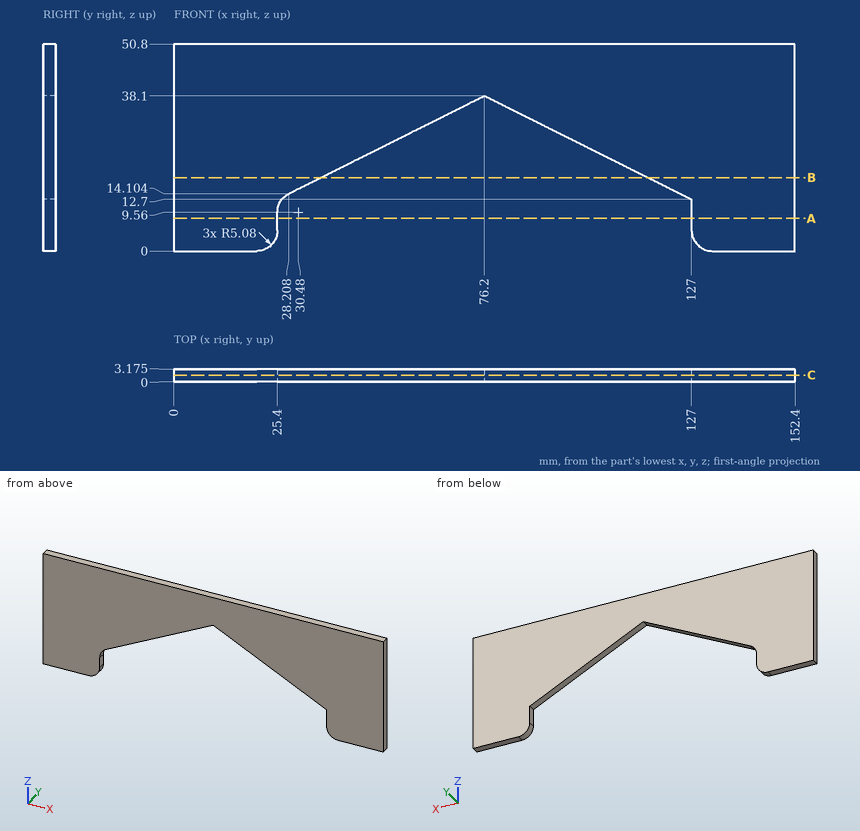
Design review of the part shown in the three views and the two pictorial views. Dimensions are in mm from the part's minimum x, y and z. Give positions to 0.01 mm unless a question says otherwise; leave off trailing zeros. Write each loop counter-clockwise with the first axis right and the second up, starting at its lowest first coordinate (ties: lowest second). Pieces come first, ordered by that corner, then holes. Notation, with made-up numbers: (53.5, 73) -> (82.5, 73) arc R15 ccw to (82.5, 83) -> close; hole circle Ø10 at (38.25, 45.25). An arc over 180 degrees is marked (long way). Answer in a Markdown table with one row per item.
1) Add section A-A on z = 8. State the section outline as (x, y) points (1 decimal).
Worked answers:
| item | result |
|---|---|
| outline | (0, 0) -> (25.4, 0) -> (25.4, 3.2) -> (0, 3.2) -> close; (127, 0) -> (152.4, 0) -> (152.4, 3.2) -> (127, 3.2) -> close |
2) Clearance check with a flat-ended pin moving along its axis: P1, Ø10, axis at x = 48, z = 19, coming from the +Y side (3 decimals). State where the tip first meets the part, or that it passes through.
Worked answers:
| item | result |
|---|---|
| P1 | y = 3.175 |
3) Add section B-B on z = 18. State the section outline as (x, y) points (1 decimal).
Worked answers:
| item | result |
|---|---|
| outline | (0, 0) -> (36, 0) -> (36, 3.2) -> (0, 3.2) -> close; (116.4, 0) -> (152.4, 0) -> (152.4, 3.2) -> (116.4, 3.2) -> close |
4) For L1, parallel to X at y = 0.5, z = 10; L2, parallel to X at y = 1.45, z = 23; L3, parallel to Z at x = 113.5, y = 2.7, list the stretches that pass through material, from the lowest coordinate up. Write a range as [from, to].
Worked answers:
| item | result |
|---|---|
| L1 | [0, 25.42], [127, 152.4] |
| L2 | [0, 46], [106.4, 152.4] |
| L3 | [19.45, 50.8] |
5) Add section C-C on y = 1.7. State the section outline as (x, z) points.
Worked answers:
| item | result |
|---|---|
| outline | (0, 0) -> (20.32, 0) arc R5.08 ccw to (25.4, 5.08) -> (25.4, 9.56) arc R5.08 cw to (28.21, 14.1) -> (76.2, 38.1) -> (127, 12.7) -> (127, 5.08) arc R5.08 ccw to (132.08, 0) -> (152.4, 0) -> (152.4, 50.8) -> (0, 50.8) -> close |
